Geometry: final body of the model. Coordinates: model frame, mm. A direction names the side the tool comes from. Coordinates: 2 decimals unless noted, no trailing zeros. Write each loop counter-clockwise with the first axis right and the second up, starting at its lowest first coordinate (ties: lowest second). Pieces come first, ordered by that corner, then holes. Notation, with made-up numbers: (45, -39) - (71, -39) arc R11 ccw to (71, -30) - close; hole circle Ø3 at (21.25, -7.75). An arc over 180 degrees is marked (long way). Put each result on its own line as item: value.
```python
from build123d import *

# Parameters (mm, degrees)
SKETCH6_W           = 66
SKETCH6_H           = 53.2
SKETCH6_R           = 1
BOSS_EXTRUDE1_DEPTH = 1.5
SKETCH7_W           = 18
SKETCH7_H           = 8
SKETCH7_W_2         = 24
SKETCH7_H_2         = 10
SKETCH7_W_3         = 11
SKETCH7_H_3         = 6
CUT_EXTRUDE1_DEPTH  = 1.5
SKETCH8_R           = 3
BOSS_EXTRUDE2_DEPTH = 5
FILLET1_R           = 1.5
SKETCH9_R           = 1.5
CUT_EXTRUDE2_DEPTH  = 487.862929815


with BuildPart() as part:
    # Sketch6 → Boss-Extrude1 (new body)
    with BuildSketch(Plane.XY.offset(10)):
        with Locations((179.113788697, 411.579190598)):
            Rectangle(SKETCH6_W, SKETCH6_H)
        with Locations((175.972708226, 433.009408695)):
            Circle(SKETCH6_R, mode=Mode.SUBTRACT)
        with Locations((181.972708226, 433.009408695)):
            Circle(SKETCH6_R, mode=Mode.SUBTRACT)
        with Locations((174.991265937, 408.983186548)):
            Circle(SKETCH6_R, mode=Mode.SUBTRACT)
        with Locations((182.991265937, 408.983186548)):
            Circle(SKETCH6_R, mode=Mode.SUBTRACT)
        with Locations((162.926862189, 435.050185267)):
            Circle(SKETCH6_R, mode=Mode.SUBTRACT)
        with Locations((194.926862189, 435.050185267)):
            Circle(SKETCH6_R, mode=Mode.SUBTRACT)
        with Locations((162.926862189, 405.077351054)):
            Circle(SKETCH6_R, mode=Mode.SUBTRACT)
        with Locations((194.926862189, 405.077351054)):
            Circle(SKETCH6_R, mode=Mode.SUBTRACT)
        with Locations((163.926862189, 387.016819786)):
            Circle(SKETCH6_R, mode=Mode.SUBTRACT)
        with Locations((193.926862189, 387.016819786)):
            Circle(SKETCH6_R, mode=Mode.SUBTRACT)
        with Locations((148.99021815, 388.016819786)):
            Circle(SKETCH6_R, mode=Mode.SUBTRACT)
        with Locations((208.935821533, 388.016819786)):
            Circle(SKETCH6_R, mode=Mode.SUBTRACT)
    extrude(amount=BOSS_EXTRUDE1_DEPTH)

    # Sketch7 → Cut-Extrude1 (cut)
    with BuildSketch(Plane.XY.offset(11.5)):
        with Locations((179.055389508, 423.939252126)):
            Rectangle(SKETCH7_W, SKETCH7_H)
        with Locations((178.85068071, 393.944335229)):
            Rectangle(SKETCH7_W_2, SKETCH7_H_2)
        with Locations((203.439714031, 400.989756962)):
            Rectangle(SKETCH7_W_3, SKETCH7_H_3)
        with Locations((154.787863363, 400.989756962)):
            Rectangle(SKETCH7_W_3, SKETCH7_H_3)
    extrude(amount=-CUT_EXTRUDE1_DEPTH, mode=Mode.SUBTRACT)

    # Sketch8 → Boss-Extrude2 (add)
    with BuildSketch(Plane.XY.offset(11.5)):
        with Locations((151.266317417, 432.621241402)):
            Circle(SKETCH8_R)
        with Locations((206.766317417, 432.621241402)):
            Circle(SKETCH8_R)
        with Locations((206.766317417, 394.121241402)):
            Circle(SKETCH8_R)
        with Locations((151.266317417, 394.121241402)):
            Circle(SKETCH8_R)
    extrude(amount=BOSS_EXTRUDE2_DEPTH)

    # Fillet1
    fillet1_edges = [part.edges().sort_by_distance(p)[0] for p in [
        (146.113788697, 438.179190598, 10.75),
        (212.113788697, 438.179190598, 10.75),
        (170.055389508, 419.939252126, 10.75),
        (212.113788697, 384.979190598, 10.75),
        (170.055389508, 427.939252126, 10.75),
        (188.055389508, 427.939252126, 10.75),
        (146.113788697, 384.979190598, 10.75),
        (188.055389508, 419.939252126, 10.75),
        (166.85068071, 388.944335229, 10.75),
        (166.85068071, 398.944335229, 10.75),
        (190.85068071, 398.944335229, 10.75),
        (190.85068071, 388.944335229, 10.75),
        (197.939714031, 397.989756962, 10.75),
        (197.939714031, 403.989756962, 10.75),
        (208.939714031, 403.989756962, 10.75),
        (208.939714031, 397.989756962, 10.75),
        (160.287863363, 403.989756962, 10.75),
        (160.287863363, 397.989756962, 10.75),
        (149.287863363, 397.989756962, 10.75),
        (149.287863363, 403.989756962, 10.75),
    ]]
    fillet(fillet1_edges, radius=FILLET1_R)

    # Sketch9 → Cut-Extrude2 (cut, through all)
    with BuildSketch(Plane.XY.offset(16.5)):
        with Locations((151.258032405, 432.638183814)):
            Circle(SKETCH9_R)
        with Locations((206.758032405, 432.638183814)):
            Circle(SKETCH9_R)
        with Locations((206.758032405, 394.138183814)):
            Circle(SKETCH9_R)
        with Locations((151.258032405, 394.138183814)):
            Circle(SKETCH9_R)
    extrude(amount=-CUT_EXTRUDE2_DEPTH, mode=Mode.SUBTRACT)


solid = part.part
```
1. Set-up query: faces 1 (the cylindrical face through (187.628, 427.488, 10.74)), 2 (the flat face through (179, 412, 11.5)), 3 (the flat face through (179, 412, 10)). Return all of +Z, -Z, +X, -X, +Y, -Y with unobstructed straight access to the full face (end or side cutting, diameter ignored); none if empty.
Answer below:
face 1: +Z, -Z
face 2: +Z
face 3: -Z, +X, -X, +Y, -Y
2. Section query D-D (y = 416.5). Return loops of the section in (x, z), then the cut area to 3 significant figures.
Answer below:
outline: (146.11, 10) - (212.11, 10) - (212.11, 11.5) - (146.11, 11.5) - close
area: 99.0 mm²
3. Section query A-A (y = 400.5). Return loops of the section in (x, z).
Answer below:
outline: (146.11, 10) - (149.29, 10) - (149.29, 11.5) - (146.11, 11.5) - close; (160.29, 10) - (197.94, 10) - (197.94, 11.5) - (160.29, 11.5) - close; (208.94, 10) - (212.11, 10) - (212.11, 11.5) - (208.94, 11.5) - close
4. Section query C-C (z = 13.75). Return loops of the section in (x, y).
Answer below:
outline: circle Ø6 at (151.27, 394.12); circle Ø6 at (151.27, 432.62); circle Ø6 at (206.77, 394.12); circle Ø6 at (206.77, 432.62); hole circle Ø3 at (151.26, 394.14); hole circle Ø3 at (151.26, 432.64); hole circle Ø3 at (206.76, 394.14); hole circle Ø3 at (206.76, 432.64)
5. Mould query, pull axis Y, two halves, no side actions, for faces 4 (the flat face through (146.114, 411, 11)), 5 (the cylindrical face through (176.43, 432.12, 10.74)), 6 (the cylindrical face through (208.14, 432.06, 13.3)), 7 (the flat face through (179, 438.179, 11)). Classes: +Y half, -Y half, draft (parallel to the pull), parting line (faces both ways), or undercut.
Answer below:
face 4: draft
face 5: undercut
face 6: undercut
face 7: +Y half
6. Section query B-B (x = 152). Return loops of the section in (y, z).
Answer below:
outline: (384.98, 10) - (392.83, 10) - (392.83, 16.5) - (391.21, 16.5) - (391.21, 11.5) - (384.98, 11.5) - close; (395.44, 10) - (397.99, 10) - (397.99, 11.5) - (397.03, 11.5) - (397.03, 16.5) - (395.44, 16.5) - close; (403.99, 10) - (431.33, 10) - (431.33, 16.5) - (429.71, 16.5) - (429.71, 11.5) - (403.99, 11.5) - close; (433.94, 10) - (438.18, 10) - (438.18, 11.5) - (435.53, 11.5) - (435.53, 16.5) - (433.94, 16.5) - close
7. Ray query, probe 1 along Y at (x, z) = (173, 10.5); probe 2 along Y at (x, z) = (201, 11); probe 3 along Y at (x, z) = (188.5, 11). Return the intervals inside material, ascending. Write a range as from..to.
Answer below:
probe 1: y = 384.98..388.94, 398.94..419.94, 427.94..438.18
probe 2: y = 384.98..397.99, 403.99..438.18
probe 3: y = 384.98..388.94, 398.94..438.18
8. Pin query (flat end, axial travel): pin 1 Ø1.5 at (x, z) = (205, 15) entering from -Y; pin 2 Ø4 at (x, y) = (187.5, 421.5) entering from +Z; pin 3 Ø3 at (x, z) = (160.5, 12) entering from +Y. Return the tip coordinate at first contact, or that it passes through.
Answer below:
pin 1: stops at y = 391.3
pin 2: stops at z = 11.5
pin 3: stops at y = 438.18
